```python
from build123d import *

# Parameters (mm, degrees)
ESQUISSE1_R                  = 5.5
BOSS_EXTRU_1_DEPTH           = 12
BOSS_EXTRU_2_DEPTH           = 6
ENL_V_MAT_EXTRU_1_DEPTH      = 16.099668871
ENL_V_MAT_EXTRU_1_DEPTH_BACK = 16.099668871
ESQUISSE3_R                  = 1.2
ESQUISSE4_R                  = 3
ENL_V_MAT_EXTRU_2_DEPTH      = 14
ESQUISSE5_R                  = 1.7
ENL_V_MAT_EXTRU_3_DEPTH      = 17.733200614


with BuildPart() as part:
    # Esquisse1 → Boss.-Extru.1 (new body)
    with BuildSketch(Plane.XY):
        Circle(ESQUISSE1_R)
    extrude(amount=BOSS_EXTRU_1_DEPTH)

    # Esquisse2 → Boss.-Extru.2 (add)
    with BuildSketch(Plane(origin=(0, 0, 0), x_dir=(-1, 0, 0), z_dir=(0, 0, -1))):
        Polygon((6, -3.464101615), (6, 3.464101615), (0, 6.92820323), (-6, 3.464101615), (-6, -3.464101615), (0, -6.92820323), align=None)
    extrude(amount=BOSS_EXTRU_2_DEPTH)

    # Esquisse3 → Enlèv. mat.-Extru.1 (cut, two sides: drawn at the far end of the back side and taken through both)
    with BuildSketch(Plane(origin=(0, 0, 0), x_dir=(0, 0, -1), z_dir=(1, 0, 0)).offset(-ENL_V_MAT_EXTRU_1_DEPTH_BACK)):
        with Locations((-8.3, 0)):
            Circle(ESQUISSE3_R)
    extrude(amount=ENL_V_MAT_EXTRU_1_DEPTH + ENL_V_MAT_EXTRU_1_DEPTH_BACK, mode=Mode.SUBTRACT)

    # Esquisse4 → Enlèv. mat.-Extru.2 (cut)
    with BuildSketch(Plane.XY.offset(12)):
        Circle(ESQUISSE4_R)
    extrude(amount=-ENL_V_MAT_EXTRU_2_DEPTH, mode=Mode.SUBTRACT)

    # Esquisse5 → Enlèv. mat.-Extru.3 (cut, through all)
    with BuildSketch(Plane.XY.offset(-2)):
        Circle(ESQUISSE5_R)
    extrude(amount=-ENL_V_MAT_EXTRU_3_DEPTH, mode=Mode.SUBTRACT)


solid = part.part
```
CAD build for the part. Positions are in the model's coordinates, mm. A direction names the side the tool comes from. Round coordinates to 2 decimals unless told otherwise and drop trailing zeros. Loops run counter-clockwise (first coordinate to the right, second up) from the corner with the lowest first, then second, coordinate; pieces in that order, holes last. Notation, with made-up numbers: M 14.25,-11.75 L 63.25,-11.75 A25 ccw 63.25,27.25 Z; hole C -17.75,5 d5. An arc over 180 degrees is marked long. Return JSON: item names as keys, results as strings. Group by question number.
(1) Wall check: probe 1 along X at (y, z) = (0, 6); probe 2 along Y at (x, z) = (-2, 8). Give the ranges that are in metal, low to high. Write a range as [from, to].
(2) Saw through at C-C, the plane z = 8.3. List the corners of the cut face in (x, y), and give its area (3 significant figures).
(3) Mould opens along Z. For faces 3 (the flat face through (6, 0, -3)), 4 (the flat face through (0, -2, -2)), 5 (the cylindrical face through (-4.14, 0.05, 9.5)) say: +Z half, -Z half, draft (parallel to the pull), parting line (faces both ways), or undercut.
(4) Saw through at B-B, the plane x = 1. List the corners of the cut face in (y, z).
(5) Saw through at A-A, the plane z = -0.75. List the corners of the cut face in (x, y), and give its area (3 significant figures).
(6) Drop flat-ended pins along their axis: P1, Ø3, axis at x = 0, y = 0, coming from the +Z side; P2, Ø4, axis at y = 0, z = 8.3, coming from the -X side; P3, Ø5, axis at x = 3, z = -4, coming from the +Y side; P4, Ø4, axis at y = -3.5, z = 2.5, coming from the -X side. Give the stop position or say it passes through.
(7) Saw through at D-D, the plane x = 4.5. List the corners of the cut face in (y, z).
(8) Tool access for faces 1 (the cylindrical face through (5.08, -2.11, 5.92)), 2 (the flat face through (-2.96, -5.22, -2.96)): list every direction of +Z, -Z, +X, -X, +Y, -Y with a clear straight run to the whole face (end or side of a thin tool).
Answer list:
{
 "1": {"probe 1": "[-5.5, -3], [3, 5.5]", "probe 2": "[-5.12, -2.24], [2.24, 5.12]"},
 "2": {"outline": "M -5.37,-1.2 A5.5 ccw 5.37,-1.2 L 2.75,-1.2 A3 cw -2.75,-1.2 Z; M -5.37,1.2 L -2.75,1.2 A3 cw 2.75,1.2 L 5.37,1.2 A5.5 ccw Z", "area": "54.6 mm2"},
 "3": {"face 3": "draft", "face 4": "+Z half", "face 5": "undercut"},
 "4": {"outline": "M -6.35,-6 L -1.37,-6 L -1.37,-2 L -2.83,-2 L -2.83,12 L -5.41,12 L -5.41,0 L -6.35,0 Z; M 1.37,-6 L 6.35,-6 L 6.35,0 L 5.41,0 L 5.41,12 L 2.83,12 L 2.83,-2 L 1.37,-2 Z"},
 "5": {"outline": "M -6,-3.46 L 0,-6.93 L 6,-3.46 L 6,3.46 L 0,6.93 L -6,3.46 Z; hole C 0,0 d6", "area": "96.4 mm2"},
 "6": {"P1": "through", "P2": "x = -5.5", "P3": "y = 6.64", "P4": "x = -5.29"},
 "7": {"outline": "M -4.33,-6 L 4.33,-6 L 4.33,0 L 3.16,0 L 3.16,12 L -3.16,12 L -3.16,0 L -4.33,0 Z; hole C 0,8.3 d2.4"},
 "8": {"face 1": "+Z", "face 2": "+Z, -Z, -X, -Y"}
}
